Model file for the job. Use its own axes, mm. Give positions to 0.01 mm unless a question says otherwise; leave off trailing zeros. Loops run counter-clockwise (first coordinate to the right, second up) from the corner with the lowest first, then second, coordinate; pieces in that order, holes last. Notation, with made-up numbers: (-28, 6) - (8, 6) arc R36 ccw to (8, 42) - close; hole circle Ø7 at (-16.5, -13). An arc over 180 degrees is marked (long way). Use a Markdown table: item, result.
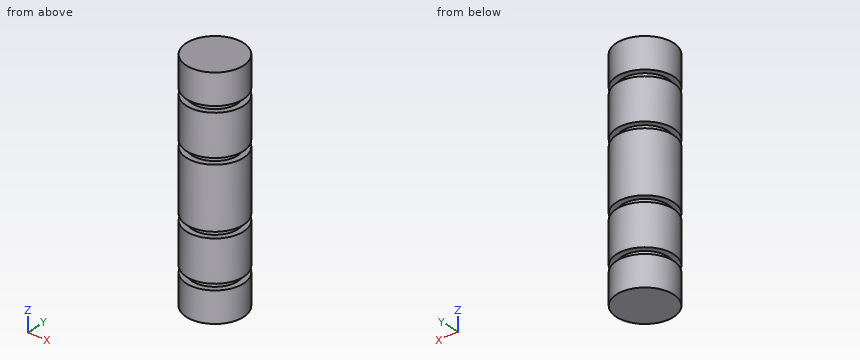
from build123d import *

# Parameters (mm, degrees)
SKETCH1_R           = 4.7625
BOSS_EXTRUDE1_DEPTH = 19.05
SKETCH2_W           = 0.9525
SKETCH2_H           = 1.016


with BuildPart() as part:
    # Sketch1 → Boss-Extrude1 (new body, symmetric)
    with BuildSketch(Plane.XY):
        Circle(SKETCH1_R)
    extrude(amount=BOSS_EXTRUDE1_DEPTH, both=True)

    # Sketch2 → Cut-Revolve1 (revolve, cut)
    with BuildSketch(Plane(origin=(0, 0, 0), x_dir=(1, 0, 0), z_dir=(0, 1, 0))):
        with Locations((4.28625, 13.462)):
            Rectangle(SKETCH2_W, SKETCH2_H)
        with Locations((4.28625, -13.462)):
            Rectangle(SKETCH2_W, SKETCH2_H)
        with Locations((4.28625, 5.588)):
            Rectangle(SKETCH2_W, SKETCH2_H)
        with Locations((4.28625, -5.588)):
            Rectangle(SKETCH2_W, SKETCH2_H)
    revolve(axis=Axis((0, 0, 19.05), (0, 0, -1)), mode=Mode.SUBTRACT)


solid = part.part
(1) Drill centre lines: probe 1 along Z at (x, y) = (3.75, -1); probe 2 along Y at (x, z) = (-1.5, -9); probe 3 along X at (y, z) = (-2.25, 2.5). Where is each one in solid material? Low to high. Write a range as [from, to].
Computed:
| item | result |
|---|---|
| probe 1 | [-19.05, -13.97], [-12.95, -6.1], [-5.08, 5.08], [6.1, 12.95], [13.97, 19.05] |
| probe 2 | [-4.52, 4.52] |
| probe 3 | [-4.2, 4.2] |
(2) Pin check, flat tips, straight feed: P1, Ø3, axis at y = -2.5, z = -6.5, coming from the +X side; P2, Ø1, axis at x = 2.5, z = 0, coming from the -Y side. Stop position of each tip, or through.
Computed:
| item | result |
|---|---|
| P1 | x = 4.66 |
| P2 | y = -4.32 |
(3) Slice it at A-A, the plane z = -11. Write the cut outline in (x, y) (1 decimal).
Computed:
| item | result |
|---|---|
| outline | circle Ø9.5 at (0, 0) |
